Geometry: final body of the model. Coordinates: model frame, mm. A direction names the side the tool comes from. Round coordinates to 2 decimals unless told otherwise and drop trailing zeros. Write each loop counter-clockwise with the first axis right and the second up, starting at its lowest first coordinate (ties: lowest second). Pieces come first, ordered by that corner, then holes.
from build123d import *


with BuildPart() as part:
    # Sketch1 → Revolve1 (revolve)
    with BuildSketch(Plane.XY, mode=Mode.PRIVATE) as revolve1_sk:
        with BuildLine():
            Line((-27.432, 15.875), (10.248650979, 5.7785))
            Line((10.248650979, 5.7785), (13.423650979, 5.7785))
            ThreePointArc((13.423650979, 5.7785), (18.15901576, 7.066472027), (21.624710712, 10.540879898))
            Line((21.624710712, 10.540879898), (27.432, 20.5994))
            Line((27.432, 20.5994), (27.432, 23.3934))
            Line((27.432, 23.3934), (27.051, 23.7744))
            Line((27.051, 23.7744), (20.4978, 23.7744))
            Line((20.4978, 23.7744), (20.4978, 25.2095))
            Line((20.4978, 25.2095), (17.3228, 25.2095))
            Line((17.3228, 25.2095), (17.3228, 22.2123))
            Line((17.3228, 22.2123), (15.5448, 22.2123))
            Line((15.5448, 22.2123), (15.5448, 20.447))
            Line((15.5448, 20.447), (14.1478, 19.05))
            Line((14.1478, 19.05), (-26.67, 19.05))
            Line((-26.67, 19.05), (-27.432, 18.288))
            Line((-27.432, 18.288), (-27.432, 15.875))
        make_face()
    revolve(revolve1_sk.sketch.rotate(Axis((-39.917319276, 0, 0), (1, 0, 0)), 90), axis=Axis((-39.917319276, 0, 0), (1, 0, 0)))


solid = part.part
1) Reachability of faces 5 (the cylindrical face through (11.86, -4.87, 3.11)), 6 (the flat face through (15.545, 6, 20)), 7 (the flat face through (20.498, -15, -19)) from +Z, -Z, +X, -X, +Y, -Y: full face, straight path, thin tool, end or side. Return the list, or none.
2) Draft query along Y for faces 1 (the flat face through (-27.432, -15, -6)), 2 (the conical face through (-4.14, -2.89, 9.19)), 3 (the conical face through (21.988, 10.904, -2.421)), 4 (the cylindrical face through (16.421, -6.672, 21.187)). Return one class per face: pulls with the +Y half, pulls with the -Y half, needs draft (parallel to the pull), parting line crosses it, or undercut.
3) Section D-D on x = -21. Output: boundary loops of the cut face in (y, z), plus the area to 3 significant figures.
4) Section C-C on x = 9. Output: boundary loops of the cut face in (y, z).
5) Line query: probe 1 along Y at (x, z) = (11, 0); probe 2 along Y at (x, z) = (0, -6); probe 3 along Z at (x, y) = (17, 3). Output: solid intervals per line, ascending.
6) First-contact query: P1, Ø15, axis at y = 0, z = 0, coming from the +X side; P2, Ø5, axis at y = -1, z = -15.5, coming from the +X side; P3, Ø10, axis at x = 6, z = -16, coming from the +Y side. Flat tips, straight axial feed; report the tip coordinate or a pass-through.
Filled in:
1. face 5: +X, -X
1. face 6: -X
1. face 7: +X
2. face 1: needs draft
2. face 2: undercut
2. face 3: undercut
2. face 4: parting line crosses it
3. outline: circle Ø38.1 at (0, 0); hole circle Ø28.3 at (0, 0)
3. area: 511 mm2
4. outline: circle Ø38.1 at (0, 0); hole circle Ø12.23 at (0, 0)
5. probe 1: y = -19.05 to -5.78, 5.78 to 19.05
5. probe 2: y = -18.08 to -6.06, 6.06 to 18.08
5. probe 3: z = -22.01 to -5.76, 5.76 to 22.01
6. P1: stops at x = 18.84
6. P2: stops at x = 25.95
6. P3: stops at y = 15.55
